Drawing for the job (mm, zero at the part's lowest x, y, z). A direction names the side the tool comes from. Round coordinates to 2 decimals unless told otherwise and drop trailing zeros. Loops run counter-clockwise (first coordinate to the right, second up) from the corner with the lowest first, then second, coordinate; pieces in that order, holes last. Notation, with made-up numbers: M 35,-21.75 L 51,-21.75 A25 ccw 51,-3.75 Z; hole C 17,-33 d9. An arc over 180 degrees is marked long. Answer in a Markdown table with one row per item.
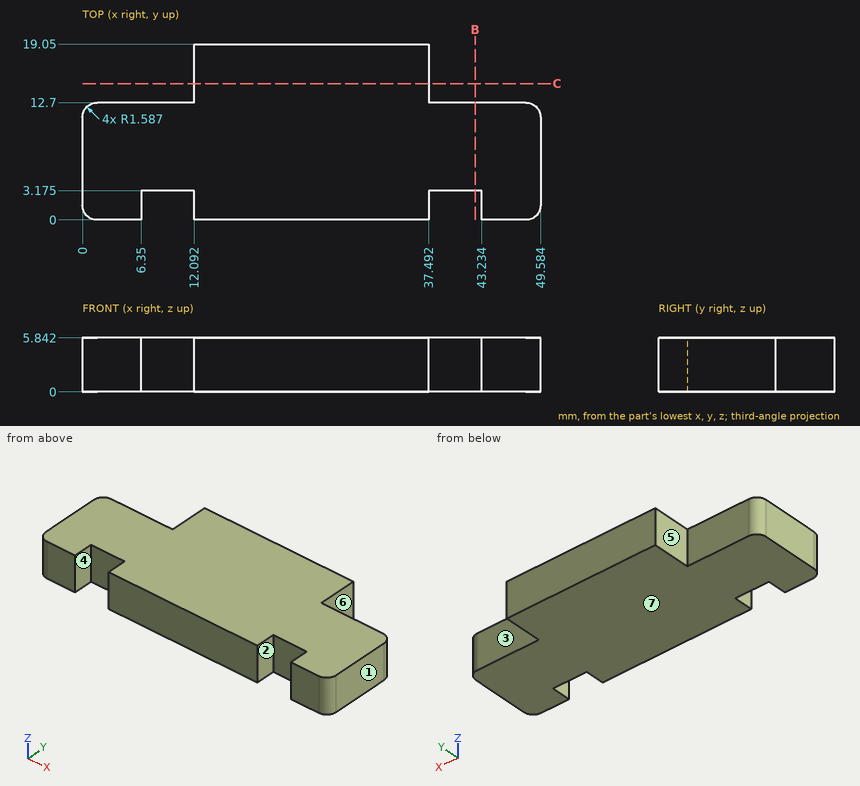
1. Mould opens along X. For the marked faces 1, 2 and 3 say: +X half, -X half, draft (parallel to the pull), parting line (faces both ways), or undercut.
Verdict:
| item | result |
|---|---|
| face 1 | +X half |
| face 2 | undercut |
| face 3 | draft |
2. Pin check, flat tips, straight feed: pin 1 (3 mm diameter, centred on x = 9.5, z = 4, fed in from -Y) (1 decimal); pin 2 (1 mm diameter, centred on y = 1, z = 1.5, fed in from +X); pin 3 (3 mm diameter, centred on x = 4.5, z = 4, fed in from +Y). Stop position of each tip, or through.
Verdict:
| item | result |
|---|---|
| pin 1 | stops at y = 3.2 |
| pin 2 | stops at x = 49.58 |
| pin 3 | stops at y = 12.7 |
3. Wall check: probe 1 along Y at (x, z) = (2.5, 5.3); probe 2 along X at (y, z) = (14, 3.65); probe 3 along Y at (x, z) = (40.5, 2.2) (1 decimal). Give the ranges that are in metal, low to high.
Verdict:
| item | result |
|---|---|
| probe 1 | y = 0 to 12.7 |
| probe 2 | x = 12.09 to 37.49 |
| probe 3 | y = 3.2 to 12.7 |
4. Saw through at C-C (y = 14.75). Write the cut outline in (x, z).
Verdict:
| item | result |
|---|---|
| outline | M 12.09,0 L 37.49,0 L 37.49,5.84 L 12.09,5.84 Z |
5. Saw through at B-B (x = 42.5). Write the cut outline in (y, z) (1 decimal).
Verdict:
| item | result |
|---|---|
| outline | M 3.2,0 L 12.7,0 L 12.7,5.8 L 3.2,5.8 Z |
6. Tool access for the marked faces 4, 5, 6 and 7: list every direction of +Z, -Z, +X, -X, +Y, -Y with a clear straight run to the whole face (end or side of a thin tool).
Verdict:
| item | result |
|---|---|
| face 4 | +Z, -Z, -Y |
| face 5 | +Z, -Z, -X, +Y |
| face 6 | +Z, -Z, +X, +Y |
| face 7 | -Z, +X, -X, +Y, -Y |
